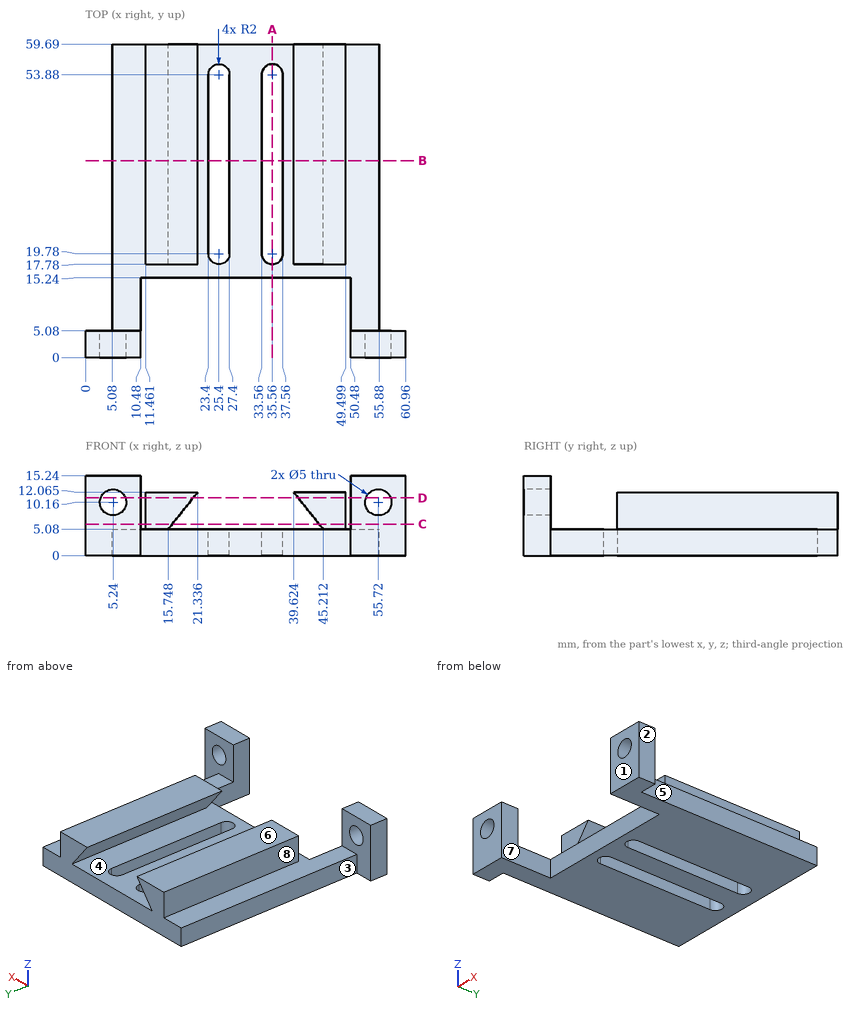
Could you check a few things on this drawing? It's one solid part, dimensions in mm from its lowest x, y, z. A direction names the side the tool comes from. Coordinates: 2 decimals unless noted, no trailing zeros. Order: outer loops, then holes, each group sorted by start corner. A loop starts at its lowest first (then second) coordinate and runs counter-clockwise, first axis right, second up. Notation, with made-up numbers: (57, 21.5) - (79, 21.5) arc R21 cw to (79, 47.5) - close; hole circle Ø4 at (-36.5, 28). An arc over 180 degrees is marked (long way). One line per question, with ' | ' between items.
(1) If I drill on L1, parallel to X at y = 2, z = 10.16; L2, parallel to Z at x = 55.72, y = 3.4; L3, parallel to Z at x = 54.5, y = 25.5, over which ranges is the centre line in solid material (lowest first)?
Report:
L1: x = 0 to 2.74, 7.74 to 10.48, 50.48 to 53.22, 58.22 to 60.96 | L2: z = 0 to 7.66, 12.66 to 15.24 | L3: z = 0 to 5.08
(2) If we mould it in two halves opening along X, with no side actions, what happens to the marked faces 1, 2, 3 and 4? For each: pulls with the +X half, pulls with the -X half, needs draft (parallel to the pull), parting line crosses it, or undercut.
Report:
face 1: needs draft | face 2: pulls with the +X half | face 3: pulls with the -X half | face 4: undercut
(3) Will these pins go through, and if not, where does the flat tip stop? pin 1 (3 mm diameter, centred on x = 9, z = 11, fed in from +Y); pin 2 (1.5 mm diameter, centred on y = 43.5, z = 2, fed in from -X); pin 3 (8 mm diameter, centred on x = 43.5, y = 29.5, fed in from +Z) (3 decimals).
Report:
pin 1: stops at y = 5.08 | pin 2: stops at x = 5.08 | pin 3: stops at z = 12.065
(4) Suppose I cut it at B-B on y = 37.5. List the corners of the cut face in (x, z) for me (1 decimal), and give its area (3 significant figures).
Report:
outline: (5.1, 0) - (23.4, 0) - (23.4, 5.1) - (15.7, 5.1) - (21.3, 12.1) - (11.5, 12.1) - (11.5, 5.1) - (5.1, 5.1) - close; (27.4, 0) - (33.6, 0) - (33.6, 5.1) - (27.4, 5.1) - close; (37.6, 0) - (55.9, 0) - (55.9, 5.1) - (49.5, 5.1) - (49.5, 12.1) - (39.6, 12.1) - (45.2, 5.1) - (37.6, 5.1) - close | area: 316 mm2
(5) Suppose I cut it at D-D on z = 11. List the corners of the cut face in (x, y) for me (1 decimal).
Report:
outline: (0, 0) - (2.9, 0) - (2.9, 5.1) - (0, 5.1) - close; (7.6, 0) - (10.5, 0) - (10.5, 5.1) - (7.6, 5.1) - close; (11.5, 17.8) - (20.5, 17.8) - (20.5, 59.7) - (11.5, 59.7) - close; (40.5, 17.8) - (49.5, 17.8) - (49.5, 59.7) - (40.5, 59.7) - close; (50.5, 0) - (53.4, 0) - (53.4, 5.1) - (50.5, 5.1) - close; (58.1, 0) - (61, 0) - (61, 5.1) - (58.1, 5.1) - close
(6) Suppose I cut it at A-A on x = 35.56. List the corners of the cut face in (y, z) for me.
Report:
outline: (15.24, 0) - (17.78, 0) - (17.78, 5.08) - (15.24, 5.08) - close; (55.88, 0) - (59.69, 0) - (59.69, 5.08) - (55.88, 5.08) - close
(7) Suppose I cut it at C-C on z = 6. List the corners of the cut face in (x, y) for me.
Report:
outline: (0, 0) - (10.48, 0) - (10.48, 5.08) - (0, 5.08) - close; (11.46, 17.78) - (16.48, 17.78) - (16.48, 59.69) - (11.46, 59.69) - close; (44.48, 17.78) - (49.5, 17.78) - (49.5, 59.69) - (44.48, 59.69) - close; (50.48, 0) - (60.96, 0) - (60.96, 5.08) - (50.48, 5.08) - close
(8) For the marked faces 5, 6, 7 and 8, which set-ups out of +Z, -Z, +X, -X, +Y, -Y let a thin tool reach every point of the face, with its end or its side?
Report:
face 5: +Z, -Z, +X, +Y | face 6: +Z, +X, -X, +Y, -Y | face 7: +Z, -Z, -Y | face 8: +Z, -X, +Y, -Y
